Design review of the part built by this model. Coordinates are the model's own, in mm. A direction names the side the tool comes from. Round coordinates to 2 decimals unless told otherwise and drop trailing zeros. Loops run counter-clockwise (first coordinate to the right, second up) from the corner with the lowest first, then second, coordinate; pieces in that order, holes last. Notation, with made-up numbers: (69.25, 10) - (117.25, 10) arc R25 cw to (117.25, 41) - close; hole circle Ø6 at (81.25, 59.5). An arc over 180 degrees is marked (long way). Return JSON: item names as keys, results as strings. Group by question number.
(1) For faces 1 (the flat face through (-36, 24, 0)), 2 (the flat face through (-26, 21.258, 1)), 3 (the flat face through (-36.43, 14.97, 4.49)), 4 (the flat face through (-29.831, 25, 1)), list the 3-axis set-ups (+Z, -Z, +X, -X, +Y, -Y) from which the entire face can be reached by the end or side of a thin tool; tool diameter is ignored.
(2) Wall thickness on L1, parallel to Y at x = -29.5, z = 4.7; L2, parallel to Y at x = -37, z = 4.5; L3, parallel to Y at x = -27, z = 4.05: over which ranges is each line inside the solid? List them lowest first. Write a range as [from, to].
(3) The part is to be moulded in two halves that separate along Y. For faces 5 (the flat face through (-27, 24, 0)), 6 (the flat face through (-34.923, 20.405, 4.493)), say which applies: pulls with the +Y half, pulls with the -Y half, needs draft (parallel to the pull), parting line crosses it, or undercut.
(4) We need section D-D, the plane x = -39. Write out the cut boundary in (y, z), and give its area (3 significant figures).
(5) We need section A-A, the plane z = 1.65. Write out the cut boundary in (x, y), and give its area (3 significant figures).
(6) We need section C-C, the plane x = -25.75. Write out the cut boundary in (y, z).
(7) Clearance check with flat-ended pins moving along their axes: pin 1 (1 mm diameter, centred on x = -35.5, y = 18, fed in from +Z); pin 2 (1.1 mm diameter, centred on x = -31, z = 4.5, fed in from -Y); pin 3 (2 mm diameter, centred on y = 15, z = 0.5, fed in from -X); pin 4 (2 mm diameter, centred on x = -27.5, z = 1, fed in from +Y). State where each tip first meets the part, or that it passes through.
(8) We need section B-B, the plane y = 22.5. Write out the cut boundary in (x, z), and give its area (3 significant figures).
from build123d import *

# Parameters (mm, degrees)
F0_R     = 9
F1_DEPTH = 4
F3_W     = 3
F3_H     = 3
F4_DEPTH = 2
F2_R     = 9
F2_R_2   = 8
F5_DEPTH = 1


with BuildPart() as f1:
    # F0 (on Top) → F1 (new body)
    with BuildSketch(Plane.XY):
        with Locations((-31.3306450844, 19.7580661625)):
            Circle(F0_R)
    extrude(amount=F1_DEPTH)

    # F3 (on face) → F4 (cut)
    with BuildSketch(Plane(origin=(0, 0, 0), x_dir=(1, 0, 0), z_dir=(0, 0, -1))):
        with BuildLine():
            ThreePointArc((-32.8306450844, -28.6321858371), (-32.0832814269, -28.7265408676), (-31.3306450844, -28.7580661625))
            ThreePointArc((-31.3306450844, -28.7580661625), (-30.5780087419, -28.7265408676), (-29.8306450844, -28.6321858371))
            Line((-29.8306450844, -28.6321858371), (-29.8306450844, -21.2580661625))
            Line((-29.8306450844, -21.2580661625), (-32.8306450844, -21.2580661625))
            Line((-32.8306450844, -21.2580661625), (-32.8306450844, -28.6321858371))
        make_face()
        with BuildLine():
            ThreePointArc((-40.204764759, -18.2580661625), (-40.2991197895, -19.0054298199), (-40.3306450844, -19.7580661625))
            ThreePointArc((-40.3306450844, -19.7580661625), (-40.2991197895, -20.510702505), (-40.204764759, -21.2580661625))
            Line((-40.204764759, -21.2580661625), (-32.8306450844, -21.2580661625))
            Line((-32.8306450844, -21.2580661625), (-32.8306450844, -18.2580661625))
            Line((-32.8306450844, -18.2580661625), (-40.204764759, -18.2580661625))
        make_face()
        with Locations((-31.3306450844, -19.7580661625)):
            Rectangle(F3_W, F3_H)
        with BuildLine():
            Line((-29.8306450844, -18.2580661625), (-29.8306450844, -21.2580661625))
            Line((-29.8306450844, -21.2580661625), (-22.4565254097, -21.2580661625))
            ThreePointArc((-22.4565254097, -21.2580661625), (-22.3621703793, -20.510702505), (-22.3306450844, -19.7580661625))
            ThreePointArc((-22.3306450844, -19.7580661625), (-22.3621703793, -19.0054298199), (-22.4565254097, -18.2580661625))
            Line((-22.4565254097, -18.2580661625), (-29.8306450844, -18.2580661625))
        make_face()
        with BuildLine():
            Line((-32.8306450844, -10.8839464878), (-32.8306450844, -18.2580661625))
            Line((-32.8306450844, -18.2580661625), (-29.8306450844, -18.2580661625))
            Line((-29.8306450844, -18.2580661625), (-29.8306450844, -10.8839464878))
            ThreePointArc((-29.8306450844, -10.8839464878), (-30.5780087419, -10.7895914574), (-31.3306450844, -10.7580661625))
            ThreePointArc((-31.3306450844, -10.7580661625), (-32.0832814269, -10.7895914574), (-32.8306450844, -10.8839464878))
        make_face()
    extrude(amount=-F4_DEPTH, mode=Mode.SUBTRACT)

    # F2 (on face) → F5 (join)
    with BuildSketch(Plane.XY.offset(4)):
        with Locations((-31.3306450844, 19.7580661625)):
            Circle(F2_R)
        with Locations((-31.3306450844, 19.7580661625)):
            Circle(F2_R_2, mode=Mode.SUBTRACT)
        Polygon((-31.5887257457, 24.8875524849), (-32.4354991317, 24.8875524849), (-32.5466804206, 22.920306772), (-37.6978889108, 21.4031711221), (-37.6978889108, 20.1682914048), (-37.0275266469, 19.7096224874), (-32.7583737671, 21.1209114641), (-32.7230915427, 17.2045808285), (-36.3218821585, 16.1813963205), (-36.6747044027, 15.3699042276), (-36.1807532609, 14.5584121346), (-34.9105931818, 14.5584121346), (-33.6051471531, 15.4404686764), (-29.2654298246, 15.4404686764), (-28.877325356, 14.9242647582), (-28.1173038363, 14.9242647582), (-27.2190589458, 16.0402674228), (-28.6656320095, 17.2045808285), (-31.5887257457, 17.2045808285), (-31.5887257457, 21.1561955512), (-29.0184542537, 21.1561955512), (-28.1363967806, 20.1330091804), (-27.0426478237, 20.1330091804), (-24.8198658228, 22.1793800592), (-31.5887257457, 22.920306772), align=None)
    extrude(amount=F5_DEPTH)


solid = f1.part
Solutions:
{
 "1": {"face 1": "-Z, +X, -X, +Y, -Y", "face 2": "-Z, +X, -X", "face 3": "+Z", "face 4": "-Z, +Y, -Y"},
 "2": {"L1": "[10.95, 11.97], [15.44, 17.2], [21.16, 22.69], [27.55, 28.57]", "L2": "[12.77, 14.11], [19.72, 21.61], [25.4, 26.75]", "L3": "[11.87, 13.03], [20.17, 22.42], [26.48, 27.65]"},
 "3": {"face 5": "needs draft", "face 6": "undercut"},
 "4": {"outline": "(15.05, 0) - (18.26, 0) - (18.26, 2) - (21.26, 2) - (21.26, 0) - (24.47, 0) - (24.47, 5) - (22.03, 5) - (22.03, 4) - (17.48, 4) - (17.48, 5) - (15.05, 5) - close", "area": "36.5 mm^2"},
 "5": {"outline": "(-40.2, 18.26) arc R9 ccw to (-32.83, 10.88) - (-32.83, 18.26) - close; (-40.2, 21.26) - (-32.83, 21.26) - (-32.83, 28.63) arc R9 ccw to start; (-29.83, 10.88) arc R9 ccw to (-22.46, 18.26) - (-29.83, 18.26) - close; (-29.83, 21.26) - (-22.46, 21.26) arc R9 ccw to (-29.83, 28.63) - close", "area": "156 mm^2"},
 "6": {"outline": "(12.7, 0) - (18.26, 0) - (18.26, 2) - (21.26, 2) - (21.26, 0) - (26.82, 0) - (26.82, 5) - (25.49, 5) - (25.49, 4) - (22.28, 4) - (22.28, 5) - (21.32, 5) - (21.32, 4) - (14.03, 4) - (14.03, 5) - (12.7, 5) - close"},
 "7": {"pin 1": "z = 4", "pin 2": "y = 10.76", "pin 3": "x = -39.51", "pin 4": "y = 28.3"},
 "8": {"outline": "(-39.9, 0) - (-32.83, 0) - (-32.83, 2) - (-29.83, 2) - (-29.83, 0) - (-22.76, 0) - (-22.76, 5) - (-23.82, 5) - (-23.82, 4) - (-27.75, 4) - (-27.75, 5) - (-33.97, 5) - (-33.97, 4) - (-38.85, 4) - (-38.85, 5) - (-39.9, 5) - close", "area": "70.9 mm^2"}
}
